```python
from build123d import *

# Parameters (mm, degrees)
SKETCH1_W           = 160
SKETCH1_H           = 52
SKETCH1_W_2         = 15
SKETCH1_H_2         = 3
BOSS_EXTRUDE1_DEPTH = 3
CUT_EXTRUDE1_DEPTH  = 3
SKETCH3_R           = 1.63582752
SKETCH3_R_2         = 1.692495787
SKETCH3_R_3         = 1.410083192
SKETCH3_R_4         = 1.550817753
CUT_EXTRUDE2_DEPTH  = 10


with BuildPart() as part:
    # Sketch1 → Boss-Extrude1 (new body)
    with BuildSketch(Plane(origin=(0, 0, 0), x_dir=(1, 0, 0), z_dir=(0, 1, 0))):
        Rectangle(SKETCH1_W, SKETCH1_H)
        with Locations((67.5, 14.5)):
            Rectangle(SKETCH1_W_2, SKETCH1_H_2, mode=Mode.SUBTRACT)
        with Locations((47.5, 14.5)):
            Rectangle(SKETCH1_W_2, SKETCH1_H_2, mode=Mode.SUBTRACT)
        with Locations((67.5, -14.5)):
            Rectangle(SKETCH1_W_2, SKETCH1_H_2, mode=Mode.SUBTRACT)
        with Locations((47.5, -14.5)):
            Rectangle(SKETCH1_W_2, SKETCH1_H_2, mode=Mode.SUBTRACT)
        with Locations((-47.5, -14.5)):
            Rectangle(SKETCH1_W_2, SKETCH1_H_2, mode=Mode.SUBTRACT)
        with Locations((-67.5, -14.5)):
            Rectangle(SKETCH1_W_2, SKETCH1_H_2, mode=Mode.SUBTRACT)
        with Locations((-47.5, 14.5)):
            Rectangle(SKETCH1_W_2, SKETCH1_H_2, mode=Mode.SUBTRACT)
        with Locations((-67.5, 14.5)):
            Rectangle(SKETCH1_W_2, SKETCH1_H_2, mode=Mode.SUBTRACT)
    extrude(amount=BOSS_EXTRUDE1_DEPTH)

    # Sketch2 → Cut-Extrude1 (cut)
    with BuildSketch(Plane(origin=(0, 3, 0), x_dir=(1, 0, 0), z_dir=(0, 1, 0))):
        with BuildLine():
            Line((-31.658505885, 2), (-8.266387648, 2))
            ThreePointArc((-8.266387648, 2), (-6.266387648, 0), (-8.266387648, -2))
            Line((-8.266387648, -2), (-31.658505885, -2))
            ThreePointArc((-31.658505885, -2), (-33.658505885, 0), (-31.658505885, 2))
        make_face()
        with BuildLine():
            Line((31.658505885, -9.856733432), (8.266387648, -9.856733432))
            ThreePointArc((8.266387648, -9.856733432), (6.266387648, -7.856733432), (8.266387648, -5.856733432))
            Line((8.266387648, -5.856733432), (31.658505885, -5.856733432))
            ThreePointArc((31.658505885, -5.856733432), (33.658505885, -7.856733432), (31.658505885, -9.856733432))
        make_face()
        with BuildLine():
            Line((-10.747740664, 17.987567994), (11.499478158, 17.987567994))
            ThreePointArc((11.499478158, 17.987567994), (13.499478158, 15.987567994), (11.499478158, 13.987567994))
            Line((11.499478158, 13.987567994), (-10.747740664, 13.987567994))
            ThreePointArc((-10.747740664, 13.987567994), (-12.747740664, 15.987567994), (-10.747740664, 17.987567994))
        make_face()
        with BuildLine():
            Line((-31.658505885, 9.620758334), (-8.266387648, 9.620758334))
            ThreePointArc((-8.266387648, 9.620758334), (-6.266387648, 7.620758334), (-8.266387648, 5.620758334))
            Line((-8.266387648, 5.620758334), (-31.658505885, 5.620758334))
            ThreePointArc((-31.658505885, 5.620758334), (-33.658505885, 7.620758334), (-31.658505885, 9.620758334))
        make_face()
        with BuildLine():
            Line((31.658505885, 5.620758334), (8.266387648, 5.620758334))
            ThreePointArc((8.266387648, 5.620758334), (6.266387648, 7.620758334), (8.266387648, 9.620758334))
            Line((8.266387648, 9.620758334), (31.658505885, 9.620758334))
            ThreePointArc((31.658505885, 9.620758334), (33.658505885, 7.620758334), (31.658505885, 5.620758334))
        make_face()
        with BuildLine():
            Line((-31.658505885, -5.856733432), (-8.266387648, -5.856733432))
            ThreePointArc((-8.266387648, -5.856733432), (-6.266387648, -7.856733432), (-8.266387648, -9.856733432))
            Line((-8.266387648, -9.856733432), (-31.658505885, -9.856733432))
            ThreePointArc((-31.658505885, -9.856733432), (-33.658505885, -7.856733432), (-31.658505885, -5.856733432))
        make_face()
        with BuildLine():
            Line((31.658505885, -2), (8.266387648, -2))
            ThreePointArc((8.266387648, -2), (6.266387648, 0), (8.266387648, 2))
            Line((8.266387648, 2), (31.658505885, 2))
            ThreePointArc((31.658505885, 2), (33.658505885, 0), (31.658505885, -2))
        make_face()
        with BuildLine():
            Line((-10.747740664, -13.987567994), (11.499478158, -13.987567994))
            ThreePointArc((11.499478158, -13.987567994), (13.499478158, -15.987567994), (11.499478158, -17.987567994))
            Line((11.499478158, -17.987567994), (-10.747740664, -17.987567994))
            ThreePointArc((-10.747740664, -17.987567994), (-12.747740664, -15.987567994), (-10.747740664, -13.987567994))
        make_face()
    extrude(amount=-CUT_EXTRUDE1_DEPTH, mode=Mode.SUBTRACT)

    # Sketch3 → Cut-Extrude2 (cut)
    with BuildSketch(Plane(origin=(0, 3, 0), x_dir=(1, 0, 0), z_dir=(0, 1, 0))):
        with Locations((34.323103301, -23.81549711)):
            Circle(SKETCH3_R)
        with Locations((-39.276258797, -23.81549711)):
            Circle(SKETCH3_R_2)
        with Locations((-45.484369153, 23.437784188)):
            Circle(SKETCH3_R_3)
        with Locations((35.235754497, 23.565498985)):
            Circle(SKETCH3_R_4)
    extrude(amount=-CUT_EXTRUDE2_DEPTH, mode=Mode.SUBTRACT)


solid = part.part
```
Could you check a few things on this model? Use its own coordinates, in mm. A direction names the side the tool comes from. Give positions to 0.01 mm unless a question says otherwise; leave off trailing zeros. Order: outer loops, then holes, each group sorted by start corner. A loop starts at its lowest first (then second) coordinate and runs counter-clockwise, first axis right, second up.
Q1. For faces 1 (the flat face through (67, 1, -16)), 2 (the flat face through (-80, 1, 0)), which set-ups out of +Z, -Z, +X, -X, +Y, -Y let a thin tool reach every point of the face, with its end or its side?
Q2. If I drill on line 1 along X through (y, z) = (2.8, -13.5); line 2 along Z through (x, y) = (10, 1.4); line 3 along Z through (x, y) = (68, 0.45), over which ranges is the centre line in solid material (lowest first)?
Q3. We'd pull the mould along Z, two halves only. Please class faces 3 (the flat face through (-68, 1, 16)), 4 (the flat face through (80, 1, 0)), 5 (the flat face through (-1, 1, 26)): +Z half, -Z half, draft (parallel to the pull), parting line (faces both ways), or undercut.
Q4. Suppose I cut it at A-A, the plane z = 0. Write out the boundary of the cut face in (x, y), and give its area (3 significant figures).
Q5. Suppose I cut it at C-C, the plane y = 2.15. Count the separate pieces of the cut face and the enclosed holes in it, and give its area (3 significant figures).
Q6. Suppose I cut it at B-B, the plane x = -49. Write out the boundary of the cut face in (y, z), and give its area (3 significant figures).
Solution:
1. face 1: +Y, -Y
1. face 2: +Z, -Z, -X, +Y, -Y
2. line 1: x = -80 to -75, -60 to -55, -40 to 40, 55 to 60, 75 to 80
2. line 2: z = -26 to -17.99, -13.99 to -9.62, -5.62 to -2, 2 to 5.86, 9.86 to 13.99, 17.99 to 26
2. line 3: z = -26 to -16, -13 to 13, 16 to 26
3. face 3: undercut
3. face 4: draft
3. face 5: +Z half
4. outline: (-80, 0) - (-33.66, 0) - (-33.66, 3) - (-80, 3) - close; (-6.27, 0) - (6.27, 0) - (6.27, 3) - (-6.27, 3) - close; (33.66, 0) - (80, 0) - (80, 3) - (33.66, 3) - close
4. area: 316 mm2
5. separate pieces: 1
5. enclosed holes: 20
5. area: 7,090 mm2
6. outline: (0, -26) - (3, -26) - (3, -16) - (0, -16) - close; (0, -13) - (3, -13) - (3, 13) - (0, 13) - close; (0, 16) - (3, 16) - (3, 26) - (0, 26) - close
6. area: 138 mm2
